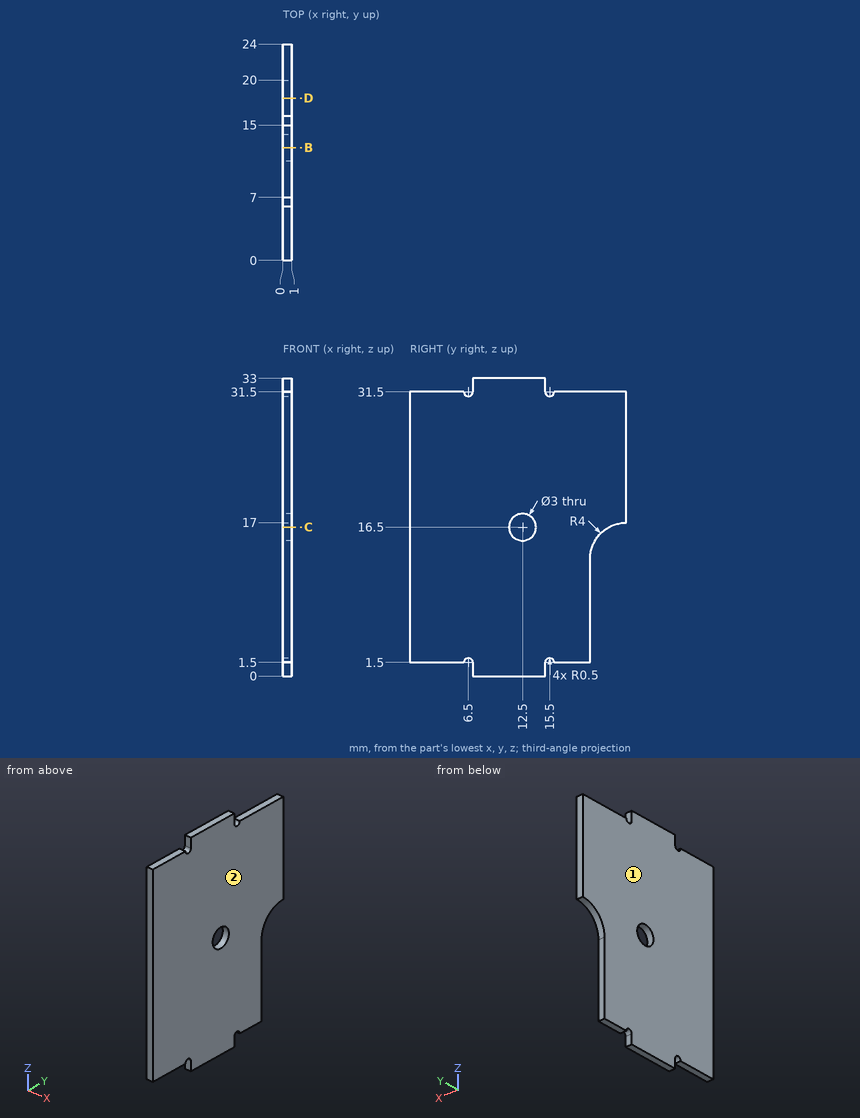
Answer from the drawing. Dimensions are ordinates in mm from the lowest x, y and z of the part. Round coordinates to 2 decimals unless told otherwise and drop trailing zeros. Write each loop counter-clockwise with the first axis right and the second up, starting at its lowest first coordinate (ties: lowest second). Pieces come first, ordered by that corner, then holes. Notation, with made-up numbers: (68, 68) - (77, 68) arc R20 ccw to (77, 95) - close; hole circle Ø2 at (29.25, -2.75). An arc over 180 degrees is marked (long way). One line per item, written item: value.
Q1. Find section B-B (y = 12.5). Determine the outline of the cut face in (x, z).
The answers:
outline: (0, 0) - (1, 0) - (1, 15) - (0, 15) - close; (0, 18) - (1, 18) - (1, 33) - (0, 33) - close
Q2. For a pull along X with two mould halves and no side action, classify the marked faces 1 and 2 as pulls with the +X half, pulls with the -X half, needs draft (parallel to the pull), parting line crosses it, or undercut.
The answers:
face 1: pulls with the -X half
face 2: pulls with the +X half
Q3. Find section C-C (z = 16.5). Determine the outline of the cut face in (x, y), and give its area (3 significant figures).
The answers:
outline: (0, 0) - (1, 0) - (1, 11) - (0, 11) - close; (0, 14) - (1, 14) - (1, 22.06) - (0, 22.06) - close
area: 19.1 mm2
Q4. Straight lines are drawn through the part: line 1 (Z direction, x = 0.6, y = 12.5); line 2 (Z direction, x = 0.9, y = 3.5); line 3 (Y direction, x = 0.4, z = 11). For each, find the intervals that lie inside material, in ascending order. Write a range as from..to.
The answers:
line 1: z = 0..15, 18..33
line 2: z = 1.5..31.5
line 3: y = 0..20
Q5. Each of these flat-tipped pins is pushed along its axis until it touches: P1, Ø2.5, axis at y = 12.5, z = 16.5, coming from the -X side; P2, Ø0.5, axis at x = 0.5, z = 32.5, coming from the -Y side; P3, Ø0.5, axis at x = 0.5, y = 4, coming from the -Z side; P4, Ø8, axis at y = 13.5, z = 8.5, coming from the -X side. Where does it stop, or does it pass through?
The answers:
P1: passes through
P2: stops at y = 7
P3: stops at z = 1.5
P4: stops at x = 0
Q6. Find section D-D (y = 18). Determine the outline of the cut face in (x, z).
The answers:
outline: (0, 1.5) - (1, 1.5) - (1, 31.5) - (0, 31.5) - close
